Autodesk Fusion 360 part; units mm, degrees
sketch "Sketch1" plane through (0, 0, 0) normal (0, 0, 1) x (1, 0, 0) in component "Base"
  line L0 (0, 0) -> (88, 0)
  line L1 (88, 0) -> (88, 60)
  line L2 (88, 60) -> (0, 60)
  line L3 (0, 60) -> (0, 0)
  line L4 (0, 11) -> (20, 11)
  line L5 (20, 11) -> (20, 49)
  line L6 (20, 49) -> (0, 49)
  line L7 (0, 49) -> (0, 11)
  circle A0 centre (23.5, 54.5) radius 1.5
  circle A1 centre (23.5, 5.5) radius 1.5
  circle A2 centre (81.5, 54.5) radius 1.5
  circle A3 centre (81.5, 5.5) radius 1.5
  line L8 (27, 49) -> (80, 49)
  line L9 (80, 49) -> (80, 11)
  line L10 (80, 11) -> (27, 11)
  line L11 (27, 11) -> (27, 49)
  line L12 (88, 48.9236) -> (83, 44)
  line L13 (83, 44) -> (83, 16)
  line L14 (83, 16) -> (88, 10.9224)
  dimension "d3" = 60
  dimension "d4" = 88
  dimension "d14" = 20
  dimension "d15" = 38
  dimension "d16" = 11
  dimension "d18" = 3
  dimension "d19" = 23.5
  dimension "d20" = 3
  dimension "d21" = 23.5
  dimension "d22" = 3
  dimension "d23" = 3
  dimension "d27" = 49
  dimension "d28" = 49
  dimension "d29" = 5.5
  dimension "d30" = 5.5
  dimension "d31" = 7
  dimension "d32" = 8
  dimension "d66" = 58
  dimension "d67" = 58
  dimension "d82" = 38
  dimension "d83" = 11
extrude "Extrude2" add sketch "Sketch1" along normal blind 6 contours L0 L1 L2 L3 L4 L5 L6 L12 L13 L14 | L1 L12 L13 L14 makes body 1 in component "Base"
extrude "Extrude1" add sketch "Sketch1" along normal blind 6 separate body contours L0 L1 L2 L3 L4 L5 L6 L12 L13 L14 | L1 L12 L13 L14 makes body 2 in component "Base"
sketch "Sketch2" plane through (0, 0, 0) normal (-1, 0, 0) x (0, -1, 0) in component "Base"
  line L0 (-60, 0) -> (-49, 0)
  line L1 (-49, 0) -> (-49, 6)
  line L2 (-49, 6) -> (-60, 6)
  line L3 (-60, 6) -> (-60, 0)
  circle A0 centre (-53.5, 3) radius 1.1
  circle A1 centre (-6.5, 3) radius 1.1
  line L4 (-11, 6) -> (0, 6)
  line L5 (0, 0) -> (0, 6)
  dimension "d35" = 2.2
  dimension "d36" = 2.2
  dimension "d37" = 3
  dimension "d38" = 3
  dimension "d39" = 47
  dimension "d40" = 6.5
extrude "Extrude3" cut sketch "Sketch2" against normal blind 18 contours A0 | A1 bodies 1 2 in component "Base"
sketch "Sketch3" plane through (0, 0, 6) normal (0, 0, 1) x (-1, 0, 0) in component "Base"
  line L0 (-80, -11) -> (-27, -11)
  line L1 (-27, -11) -> (-27, -49)
  line L2 (-27, -49) -> (-80, -49)
  line L3 (-80, -49) -> (-80, -11)
  circle A0 centre (-81.5, -54.5) radius 1.5
  circle A1 centre (-81.5, -5.5) radius 1.5
  circle A2 centre (-23.5, -5.5) radius 1.5
  circle A3 centre (-23.5, -54.5) radius 1.5
  line L4 (0, -11) -> (0, 0)
  line L5 (0, 0) -> (-88, 0)
  line L6 (-88, 0) -> (-88, -60)
  line L7 (-88, -60) -> (0, -60)
  line L8 (0, -60) -> (0, -49)
  line L9 (0, -49) -> (-20, -49)
  line L10 (-20, -49) -> (-20, -11)
  line L11 (-20, -11) -> (0, -11)
  circle A4 centre (-23.5, -54.5) radius 3.5
  circle A5 centre (-81.5, -54.5) radius 3.5
  circle A6 centre (-81.5, -5.5) radius 3.5
  circle A7 centre (-23.5, -5.5) radius 3.5
  dimension "d43" = 7
  dimension "d45" = 7
  dimension "d46" = 7
  dimension "d47" = 7
extrude "Extrude4" add sketch "Sketch3" along normal blind 2.5 contours A4 | A5 | A6 | A7 bodies 1 2 in component "Base"
sketch "Sketch4" plane through (0, 0, 0) normal (0, 0, 1) x (1, 0, 0) in component "Base"
  circle A0 centre (23.5, 5.5) radius 2.75
  circle A1 centre (81.5, 5.5) radius 2.75
  circle A2 centre (81.5, 54.5) radius 2.75
  circle A3 centre (23.5, 54.5) radius 2.75
  dimension "d51" = 5.5
  dimension "d52" = 5.5
  dimension "d53" = 5.5
  dimension "d54" = 5.5
  dimension "d77" = 58
  dimension "d78" = 58
  dimension "d79" = 49
  dimension "d80" = 49
extrude "Extrude5" cut sketch "Sketch4" along normal blind 4 bodies 1 in component "Base"
fillet "Fillet9" radius 3 12 edges at (80, 49, 3) (80, 49, 3) (20, 49, 3) (20, 49, 3) (80, 11, 3) (80, 11, 3) (20, 11, 3) (20, 11, 3) (27, 49, 3) (27, 49, 3) (27, 11, 3) (27, 11, 3) on bodies 1 2 in component "Base"
chamfer "Chamfer5" distance 1.2 angle 45 13 edges at (27, 30, 0) (27.8787, 48.1213, 0) (53.5, 49, 0) (79.1213, 48.1213, 0) (80, 30, 0) (79.1213, 11.8787, 0) (53.5, 11, 0) (27.8787, 11.8787, 0) (8.5, 11, 0) (19.1213, 11.8787, 0) (20, 30, 0) (19.1213, 48.1213, 0) (8.5, 49, 0) on bodies 1 in component "Base"
fillet "Fillet12" radius 1.2 13 edges at (79.1213, 48.1213, 6) (80, 30, 6) (79.1213, 11.8787, 6) (53.5, 11, 6) (27.8787, 11.8787, 6) (27, 30, 6) (27.8787, 48.1213, 6) (53.5, 49, 6) (8.5, 49, 6) (19.1213, 48.1213, 6) (20, 30, 6) (19.1213, 11.8787, 6) (8.5, 11, 6) on bodies 1 in component "Base"
extrude "Extrude6" cut sketch "Sketch1" along normal up to surface (6 mm away) contours L1 L12 L13 L14 bodies 1 in component "Base"
fillet "Fillet13" radius 6.5 2 edges at (83, 44, 3) (83, 16, 3) on bodies 1 in component "Base"
fillet "Fillet14" radius 3 6 edges at (88, 48.9236, 3) (88, 10.9224, 3) (88, 0, 3) (88, 0, 3) (88, 60, 3) (88, 60, 3) on bodies 1 2 in component "Base"
fillet "Fillet15" radius 1.2 13 edges at (42.5, 0, 6) (87.1213, 0.8787, 6) (88, 6.3466, 6) (87.776, 10.8307, 6) (86.0031, 12.9503, 6) (83.4853, 16.1988, 6) (83, 29.9707, 6) (83.5044, 43.7888, 6) (86.0221, 46.9759, 6) (87.7672, 49.0211, 6) (88, 53.5899, 6) (87.1213, 59.1213, 6) (42.5, 60, 6) on bodies 1 in component "Base"
chamfer "Chamfer8" distance 1 angle 45 14 edges at (0, 49, 3) (0, 49.3515, 5.6485) (0, 54.5, 6) (0, 59.6485, 5.6485) (0, 60, 2.4) (0, 55.1, 0) (0, 49.6, 0.6) (0, 11, 3) (0, 10.6485, 5.6485) (0, 5.5, 6) (0, 0.3515, 5.6485) (0, 0, 2.4) (0, 10.4, 0.6) (0, 4.9, 0) on bodies 1 in component "Base"
component "Base" placed x (1, 0, 0) y (0, 1, 0) z (0, 0, 1) at (0, 0, 0)
equation "width = 82 mm + 6 mm"
equation "height = 60 mm"
equation "d3 = height"
equation "d4 = width"
equation "firstHolesXOffset = 23.5 mm"
equation "secondHolesXOffset = 82 mm"
equation "panelHolesDistance = 47 mm"
equation "piScrewHoleDiameter = 3 mm"
equation "piScrewHeadHoleDiameter = 5.5 mm"
equation "piHoleSpacerDistance = 2.5 mm"
equation "thickness = 6 mm"
equation "d12 = thickness"
equation "d15 = cutoutHeight"
equation "d16 = ( height - cutoutHeight ) / 2"
equation "cutoutHeight = 38 mm"
equation "d18 = piScrewHoleDiameter"
equation "d19 = firstHolesXOffset"
equation "d20 = piScrewHoleDiameter"
equation "d21 = firstHolesXOffset"
equation "d22 = piScrewHoleDiameter"
equation "d23 = piScrewHoleDiameter"
equation "piHolesVerticalSpacing = 49 mm"
equation "d27 = piHolesVerticalSpacing"
equation "d28 = piHolesVerticalSpacing"
equation "d29 = ( height - piHolesVerticalSpacing ) / 2"
equation "d30 = ( height - piHolesVerticalSpacing ) / 2"
equation "d33 = thickness"
equation "d37 = thickness / 2"
equation "d38 = thickness / 2"
equation "d39 = panelHolesDistance"
equation "d40 = ( height - panelHolesDistance ) / 2"
equation "d43 = piSpacerDiameter"
equation "piSpacerDiameter = 7 mm"
equation "d45 = piSpacerDiameter"
equation "d46 = piSpacerDiameter"
equation "d47 = piSpacerDiameter"
equation "d48 = piHoleSpacerDistance"
equation "screwHeadSinkDepth = 4 mm"
equation "d51 = piScrewHeadHoleDiameter"
equation "d52 = piScrewHeadHoleDiameter"
equation "d53 = piScrewHeadHoleDiameter"
equation "d54 = piScrewHeadHoleDiameter"
equation "d55 = screwHeadSinkDepth"
equation "d82 = cutoutHeight"
equation "d83 = ( height - cutoutHeight ) / 2"
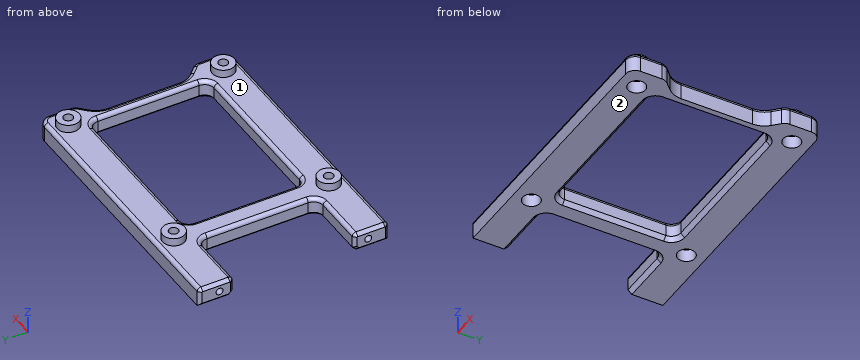
Can you work these out from the model? Positions are in its coordinate system, mm. Face numbers are marked on the shaded views. Give positions to 0.01 mm unless a question says otherwise; leave off trailing zeros. Loops run counter-clockwise (first coordinate to the right, second up) from the corner with the lowest first, then second, coordinate; pieces in that order, holes last. Notation, with made-up numbers: M -33,13.5 L -7,13.5 A29 ccw -7,50.5 Z; hole C 13.5,61 d8. An arc over 180 degrees is marked long. Answer in a Markdown table with one row per item.
1. For pin 1 Ø5 at (x, y) = (81.5, 5.5) entering from -Z; pin 2 Ø4 at (y, z) = (39, 6.5) entering from -X; pin 3 Ø2.5 at (x, y) = (23.5, 5.5) entering from -Z; pin 4 Ø1.8 at (y, z) = (37.5, 3) entering from +X, each with a flat end and sliding along its axis, tell me the tip position at first contact or that it passes through.
Taken from the geometry:
| item | result |
|---|---|
| pin 1 | stops at z = 4 |
| pin 2 | stops at x = 20 |
| pin 3 | passes through |
| pin 4 | stops at x = 83 |
2. If I drill on line 1 along Y through (x, z) = (81.5, 1.75); line 2 along X through (y, z) = (54.5, 6.8); line 3 along Z through (x, y) = (5.5, 6.5), over which ranges is the centre line in solid material (lowest first)?
Taken from the geometry:
| item | result |
|---|---|
| line 1 | y = 0 to 2.75, 8.25 to 51.75, 57.25 to 60 |
| line 2 | x = 20 to 22, 25 to 27, 78 to 80, 83 to 85 |
| line 3 | z = 0 to 1.9, 4.1 to 6 |
3. Thinking about a two-plate mould opening in X: for the marked faces 1 and 2, which applies, released by +X, released by -X, zero draft, split by the parting line, or undercut?
Taken from the geometry:
| item | result |
|---|---|
| face 1 | undercut |
| face 2 | zero draft |
4. Suppose I cut it at A-A on y = 26.5. Write out the boundary of the cut face in (x, z), plus the area to 3 significant figures.
Taken from the geometry:
| item | result |
|---|---|
| outline | M 20,1.2 L 21.2,0 L 25.8,0 L 27,1.2 L 27,4.8 A1.2 ccw 25.8,6 L 21.2,6 A1.2 ccw 20,4.8 Z; M 80,1.2 L 81.2,0 L 83,0 L 83,4.8 A1.2 ccw 81.8,6 L 81.2,6 A1.2 ccw 80,4.8 Z |
| area | 56.6 mm² |
5. Suppose I cut it at B-B on x = 31. Write out the boundary of the cut face in (y, z).
Taken from the geometry:
| item | result |
|---|---|
| outline | M 0,0 L 9.8,0 L 11,1.2 L 11,4.8 A1.2 ccw 9.8,6 L 1.2,6 A1.2 ccw 0,4.8 Z; M 49,1.2 L 50.2,0 L 60,0 L 60,4.8 A1.2 ccw 58.8,6 L 50.2,6 A1.2 ccw 49,4.8 Z |
